The drawing under review shows one solid part. Ordinate dimensions are in mm from its lowest x, y, z. A direction names the side the tool comes from. Coordinates: 2 decimals unless noted, no trailing zeros. Write each loop counter-clockwise with the first axis right and the second up, starting at its lowest first coordinate (ties: lowest second). Pieces come first, ordered by that corner, then holes.
Q1. Machinability: for the marked faces 4 and 5, which of the approach directions +Z, -Z, +X, -X, +Y, -Y give a long, thin tool a straight path to every point of the face, cutting with its end or side? Answer none if there is none.
Q2. For probe 1 along Z at (x, y) = (5, 1.35); probe 2 along X at (y, z) = (7, 10); probe 3 along Z at (x, y) = (5, 6.6), list the stretches that pass through material, from the lowest coordinate up.
Q3. Take a section at D-D (x = 8). Give the boundary of the cut face in (y, z).
Q4. Take a section at B-B (z = 10). Give the boundary of the cut face in (x, y).
Q5. Take a section at A-A (x = 5). Give the boundary of the cut face in (y, z).
Q6. Take a section at C-C (y = 5). Give the boundary of the cut face in (x, z), and give its area (3 significant figures).
Q7. Mouldability with a two-part tool opening along X and no side actions: class the marked faces 1, 2 and 3 as pulls with the +X half, pulls with the -X half, needs draft (parallel to the pull), parting line crosses it, or undercut.
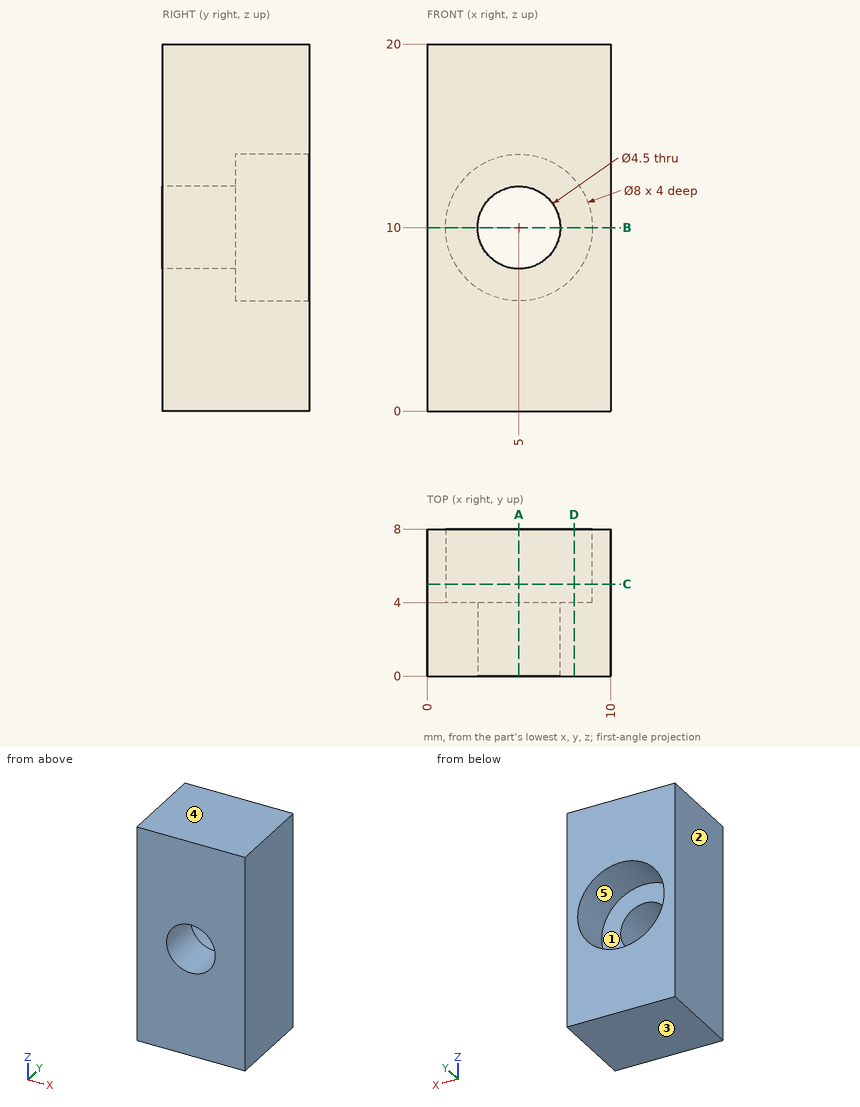
Response:
1. face 4: +Z, +X, -X, +Y, -Y
1. face 5: +Y
2. probe 1: z = 0 to 7.75, 12.25 to 20
2. probe 2: x = 0 to 1, 9 to 10
2. probe 3: z = 0 to 6, 14 to 20
3. outline: (0, 0) - (8, 0) - (8, 7.35) - (4, 7.35) - (4, 12.65) - (8, 12.65) - (8, 20) - (0, 20) - close
4. outline: (0, 0) - (2.75, 0) - (2.75, 4) - (1, 4) - (1, 8) - (0, 8) - close; (7.25, 0) - (10, 0) - (10, 8) - (9, 8) - (9, 4) - (7.25, 4) - close
5. outline: (0, 0) - (8, 0) - (8, 6) - (4, 6) - (4, 7.75) - (0, 7.75) - close; (0, 12.25) - (4, 12.25) - (4, 14) - (8, 14) - (8, 20) - (0, 20) - close
6. outline: (0, 0) - (10, 0) - (10, 20) - (0, 20) - close; hole circle Ø8 at (5, 10)
6. area: 150 mm2
7. face 1: undercut
7. face 2: pulls with the -X half
7. face 3: needs draft
